Source: CAD feature listing. Evaluate the final solid. Frame: model axes, mm. A direction names the side the tool comes from. Coordinates: 2 decimals unless noted, no trailing zeros. Order: outer loops, then holes, each group sorted by start corner. A loop starts at its lowest first (then second) coordinate and runs counter-clockwise, first axis right, second up.
```python
from build123d import *

# Parameters (mm, degrees)
BOSS_EXTRUDE1_DEPTH = 2
SKETCH1_3_R         = 4.2
SKETCH1_3_R_2       = 2.9
BOSS_EXTRUDE2_DEPTH = 5
SKETCH1_4_R         = 2.9
SKETCH1_4_R_2       = 1.5
BOSS_EXTRUDE3_DEPTH = 1.5


with BuildPart() as part:
    # Sketch1 → Boss-Extrude1 (new body)
    with BuildSketch(Plane.XY):
        with BuildLine():
            Line((4.117050837, 0.83059762), (2.325, 18.775))
            ThreePointArc((2.325, 18.775), (0, 21.1), (-2.325, 18.775))
            Line((-2.325, 18.775), (-4.117050837, 0.83059762))
            ThreePointArc((-4.117050837, 0.83059762), (0, 4.2), (4.117050837, 0.83059762))
        make_face()
    extrude(amount=BOSS_EXTRUDE1_DEPTH)

    # Sketch1_3 → Boss-Extrude2 (add)
    with BuildSketch(Plane.XY):
        Circle(SKETCH1_3_R)
        Circle(SKETCH1_3_R_2, mode=Mode.SUBTRACT)
    extrude(amount=BOSS_EXTRUDE2_DEPTH)

    # Sketch1_4 → Boss-Extrude3 (add)
    with BuildSketch(Plane.XY):
        Circle(SKETCH1_4_R)
        Circle(SKETCH1_4_R_2, mode=Mode.SUBTRACT)
    extrude(amount=BOSS_EXTRUDE3_DEPTH)


solid = part.part
```
1. Access query for faces 1 (the flat face through (0, 9, 0)), 2 (the cylindrical face through (-0.91, -4.1, 3.02)). Directions: +Z, -Z, +X, -X, +Y, -Y. A direction counts if a zero-diameter tool reaches every point of the face in a straight line with its end or side. Return the directions, or none.
2. Draft query along X for faces 3 (the flat face through (3.234, 9.677, 0.986)), 4 (the flat face through (1.2, -1.2, 1.5)), 5 (the flat face through (-3.21, 9.93, 0.99)), 6 (the flat face through (0, 11, 2)). Return one class per face: +X half, -X half, draft (parallel to the pull), parting line (faces both ways), or undercut.
3. Section query A-A, the plane y = 0. Output: boundary loops of the cut face in (x, z), plus the area to 3 significant figures.
4. Material intervals for line 1 along Y through (x, z) = (0, 1.05); line 2 along Y through (x, z) = (0, 2.9); line 3 along Z through (x, y) = (-1.5, 4.75), sorted ascending.
5. Section query B-B, the plane x = 0. Output: boundary loops of the cut face in (y, z).
6. Contact query for flat-ended pins moving along their axis: P1, Ø2.5, axis at x = 1.5, y = 9, coming from the +Z side; P2, Ø1, axis at y = 11.5, z = 4, coming from the -X side; P3, Ø3.5, axis at x = 0, y = 0, coming from the +Z side; P4, Ø1, axis at y = 3, z = 1.5, coming from the -X side. Output: stop coordinate, or through.
7. Section query D-D, the plane x = 1.25. Output: boundary loops of the cut face in (y, z).
8. Section query C-C, the plane z = 0.6. Output: boundary loops of the cut face in (x, y) (3 decimals).
Answer key:
1. face 1: -Z, +X, -X, +Y, -Y
1. face 2: +Z
2. face 3: +X half
2. face 4: undercut
2. face 5: -X half
2. face 6: draft
3. outline: (-4.2, 0) - (-1.5, 0) - (-1.5, 1.5) - (-2.9, 1.5) - (-2.9, 5) - (-4.2, 5) - close; (1.5, 0) - (4.2, 0) - (4.2, 5) - (2.9, 5) - (2.9, 1.5) - (1.5, 1.5) - close
3. area: 17.2 mm2
4. line 1: y = -4.2 to -1.5, 1.5 to 21.1
4. line 2: y = -4.2 to -2.9, 2.9 to 4.2
4. line 3: z = 0 to 2
5. outline: (-4.2, 0) - (-1.5, 0) - (-1.5, 1.5) - (-2.9, 1.5) - (-2.9, 5) - (-4.2, 5) - close; (1.5, 0) - (21.1, 0) - (21.1, 2) - (4.2, 2) - (4.2, 5) - (2.9, 5) - (2.9, 1.5) - (1.5, 1.5) - close
6. P1: stops at z = 2
6. P2: passes through
6. P3: stops at z = 1.5
6. P4: stops at x = -3.95
7. outline: (-4.01, 0) - (-0.83, 0) - (-0.83, 1.5) - (-2.62, 1.5) - (-2.62, 5) - (-4.01, 5) - close; (0.83, 0) - (20.74, 0) - (20.74, 2) - (4.01, 2) - (4.01, 5) - (2.62, 5) - (2.62, 1.5) - (0.83, 1.5) - close
8. outline: (-4.117, 0.831) arc R4.2 ccw (long way) to (4.117, 0.831) - (2.325, 18.775) arc R2.325 ccw to (-2.325, 18.775) - close; hole circle Ø3 at (0, 0)
